```python
from build123d import *

# Parameters (mm, degrees)
SKETCH1_R         = 17.526
EXTRUDE1_DEPTH    = 6.35
EXTRUDE2_START    = 6.35
SKETCH1_3_R       = 47.625
EXTRUDE2_DEPTH    = 14.224
EXTRUDE3_START    = 20.574
SKETCH1_4_R       = 19.05
EXTRUDE3_DEPTH    = 8.128
EXTRUDE4_START    = 6.35
SKETCH1_5_R       = 7.874
EXTRUDE4_DEPTH    = 14.224
CIRPATTERN1_COUNT = 4
SKETCH3_R         = 11.176
EXTRUDE5_DEPTH    = 9.652
EXTRUDE6_REACH    = 30.702
SKETCH3_3_R       = 6.9342


with BuildPart() as part:
    # Sketch1 → Extrude1 (new body)
    with BuildSketch(Plane.XY):
        Circle(SKETCH1_R)
    extrude(amount=EXTRUDE1_DEPTH)

    # Sketch1<3> → Extrude2 (add)
    with BuildSketch(Plane.XY.offset(EXTRUDE2_START)):
        Circle(SKETCH1_3_R)
    extrude(amount=EXTRUDE2_DEPTH)

    # Sketch1<4> → Extrude3 (add)
    with BuildSketch(Plane.XY.offset(EXTRUDE3_START)):
        Circle(SKETCH1_4_R)
    extrude(amount=EXTRUDE3_DEPTH)

    # Sketch1<5> → Extrude4 (cut)
    with BuildSketch(Plane.XY.offset(EXTRUDE4_START)):
        with Locations((0, 33.3375)):
            Circle(SKETCH1_5_R)
    extrude4 = extrude(amount=EXTRUDE4_DEPTH, mode=Mode.SUBTRACT)

    # CirPattern1: Extrude4 ×4 about axis
    cirpattern1_axis = Axis((0, 0, 0), (0, 0, 1))
    for i in range(1, CIRPATTERN1_COUNT):
        add(extrude4.rotate(cirpattern1_axis, i * 360 / CIRPATTERN1_COUNT), mode=Mode.SUBTRACT)

    # Sketch3 → Extrude5 (cut)
    with BuildSketch(Plane(origin=(0, 0, 28.702), x_dir=(-1, 0, 0), z_dir=(0, 0, -1))):
        Circle(SKETCH3_R)
    extrude(amount=EXTRUDE5_DEPTH, mode=Mode.SUBTRACT)

    # Sketch3<3> → Extrude6 (cut, up to next)
    with BuildSketch(Plane(origin=(0, 0, 28.702), x_dir=(-1, 0, 0), z_dir=(0, 0, -1)), mode=Mode.PRIVATE) as extrude6_sk1:
        Circle(SKETCH3_3_R)
    extrude6_tool1 = extrude(extrude6_sk1.sketch, amount=EXTRUDE6_REACH, mode=Mode.PRIVATE) & part.part
    add(extrude6_tool1.solids().sort_by_distance((0, 0, 28.702))[0], mode=Mode.SUBTRACT)


solid = part.part
```
Can you work these out from the model? Positions are in its coordinate system, mm. A direction names the side the tool comes from. Give positions to 0.01 mm unless a question says otherwise; leave off trailing zeros. Order: outer loops, then holes, each group sorted by start corner. A loop starts at its lowest first (then second) coordinate and runs counter-clockwise, first axis right, second up. Notation, with made-up numbers: M 70,14 L 117,14 A25 cw 117,45 Z; hole C 67.5,43.5 d5. An arc over 180 degrees is marked long. One line per item, written item: value.
1) On a 3-axis mill with a long thin cutter (end or side, diameter ignored), from which of +Z, -Z, +X, -X, +Y, -Y can I reach the whole of each face in a straight line? I mean faces 4 (the face through (-1.025, 41.144, 13.362)), 5 (the face through (20, 1, 20.574)), 6 (the face through (16.72, 5.26, 3.13)). Say none if no direction works.
Answer sheet:
face 4: +Z, -Z
face 5: +Z
face 6: -Z
2) We'd pull the mould along X, two halves only. Please class faces 1 (the face through (-41.144, -1.025, 13.362)), 2 (the face through (20, 1, 6.35)), 3 (the face through (-15.12, -11.59, 24.58)): released by +X, released by -X, zero draft, split by the parting line, or undercut.
Answer sheet:
face 1: undercut
face 2: zero draft
face 3: split by the parting line
3) Please list where these lines run through material, in increasing order: line 1 along Y through (x, z) = (0, 14.5) (1 decimal); line 2 along Y through (x, z) = (-6, 17.5); line 3 along Z through (x, y) = (-21.5, -24).
Answer sheet:
line 1: y = -47.6 to -41.2, -25.5 to -6.9, 6.9 to 25.5, 41.2 to 47.6
line 2: y = -47.25 to -38.44, -28.24 to -3.48, 3.48 to 28.24, 38.44 to 47.25
line 3: z = 6.35 to 20.57
4) I want a section at D-D, the plane x = 36.5. List the corners of the cut face in (y, z) for me.
Answer sheet:
outline: M -30.59,6.35 L -7.21,6.35 L -7.21,20.57 L -30.59,20.57 Z; M 7.21,6.35 L 30.59,6.35 L 30.59,20.57 L 7.21,20.57 Z
5) I want a section at C-C, the plane y = 37. List the corners of the cut face in (x, z) for me.
Answer sheet:
outline: M -29.99,6.35 L -6.97,6.35 L -6.97,20.57 L -29.99,20.57 Z; M 6.97,6.35 L 29.99,6.35 L 29.99,20.57 L 6.97,20.57 Z
6) For P1, Ø18, axis at x = -33.34, y = 0, coming from the +Z side; P2, Ø6, axis at y = 14.5, z = 7.5, coming from the -X side; P3, Ø5, axis at y = 19, z = 21.5, coming from the -X side; P4, Ø12, axis at x = -5.5, y = -2.5, coming from the +Z side, each with a flat end and sliding along its axis, tell me the tip position at first contact or that it passes through.
Answer sheet:
P1: stops at z = 20.57
P2: stops at x = -46.22
P3: stops at x = -44.61
P4: stops at z = 28.7
7) I want a section at A-A, the plane y = 0. Count the separate pieces of the cut face and the enclosed holes in it, plus the area to 3 significant figures.
Answer sheet:
separate pieces: 4
enclosed holes: 0
area: 959 mm^2
